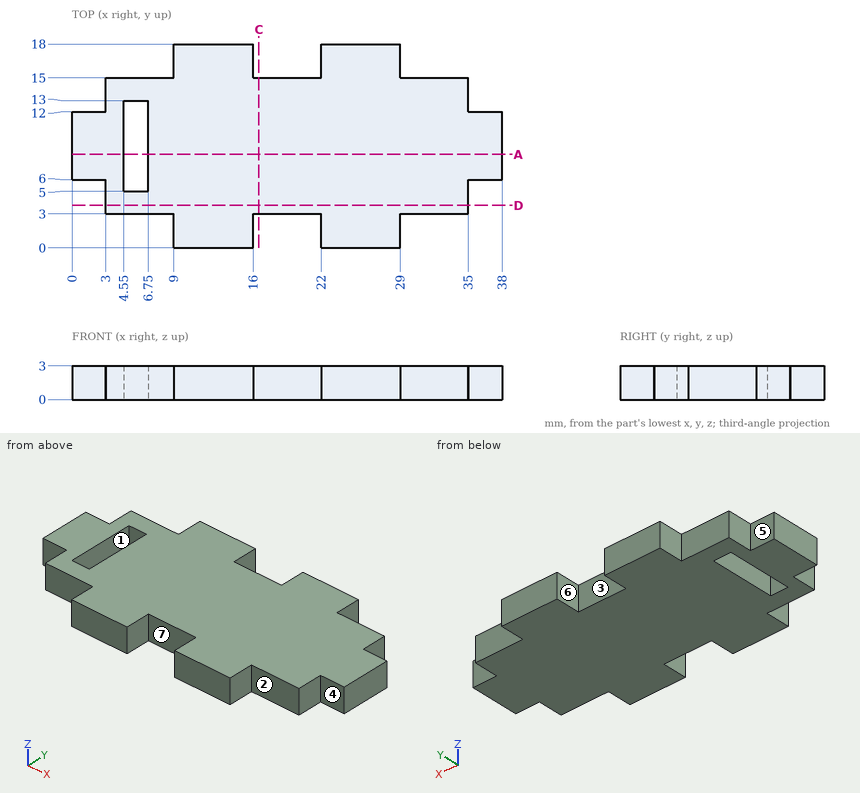
Answer from the drawing. Dimensions are ordinates in mm from the lowest x, y and z of the part. A direction names the side the tool comes from. Coordinates: 2 decimals unless noted, no trailing zeros. Loops run counter-clockwise (first coordinate to the right, second up) from the corner with the lowest first, then second, coordinate; pieces in that order, holes last.
Q1. The part is cut by section A-A on y = 8.25. Write down the section's boundary in (x, z).
Q2. Which of the six approach directions +Z, -Z, +X, -X, +Y, -Y give full straight-line access (tool end or side, diameter ignored) to the marked faces 4, 5, 6 and 7?
Q3. The mould has two halves that part along Y. Classify the marked faces 1, 2 and 3: +Y half, -Y half, draft (parallel to the pull), parting line (faces both ways), or undercut.
Q4. The part is cut by section C-C on x = 16.5. Write down the section's boundary in (y, z), and give its area (3 significant figures).
Q5. The part is cut by section D-D on y = 3.75. Write down the section's boundary in (x, z), and give its area (3 significant figures).
Q6. Consider probe 1 along X at (y, z) = (1, 1.6); probe 2 along X at (y, z) = (7.5, 1.1); probe 3 along Y at (x, z) = (8, 2.3). Determine where each line is inside the solid, lowest interval first.
Q7. Each of these flat-tipped pins is pushed along its axis until it touches: pin 1 Ø1.5 at (x, z) = (2, 1) entering from -Y; pin 2 Ø1.5 at (y, z) = (1.5, 2) entering from -X; pin 3 Ø1.1 at (x, z) = (6, 1) entering from -Y. Where does it stop, or does it pass through?
Results below:
1. outline: (0, 0) - (4.55, 0) - (4.55, 3) - (0, 3) - close; (6.75, 0) - (38, 0) - (38, 3) - (6.75, 3) - close
2. face 4: +Z, -Z, +X, -Y
2. face 5: +Z, -Z, -X, +Y
2. face 6: +Z, -Z, +Y
2. face 7: +Z, -Z, -Y
3. face 1: undercut
3. face 2: -Y half
3. face 3: +Y half
4. outline: (3, 0) - (15, 0) - (15, 3) - (3, 3) - close
4. area: 36.0 mm2
5. outline: (3, 0) - (35, 0) - (35, 3) - (3, 3) - close
5. area: 96.0 mm2
6. probe 1: x = 9 to 16, 22 to 29
6. probe 2: x = 0 to 4.55, 6.75 to 38
6. probe 3: y = 3 to 15
7. pin 1: stops at y = 6
7. pin 2: stops at x = 9
7. pin 3: stops at y = 3
